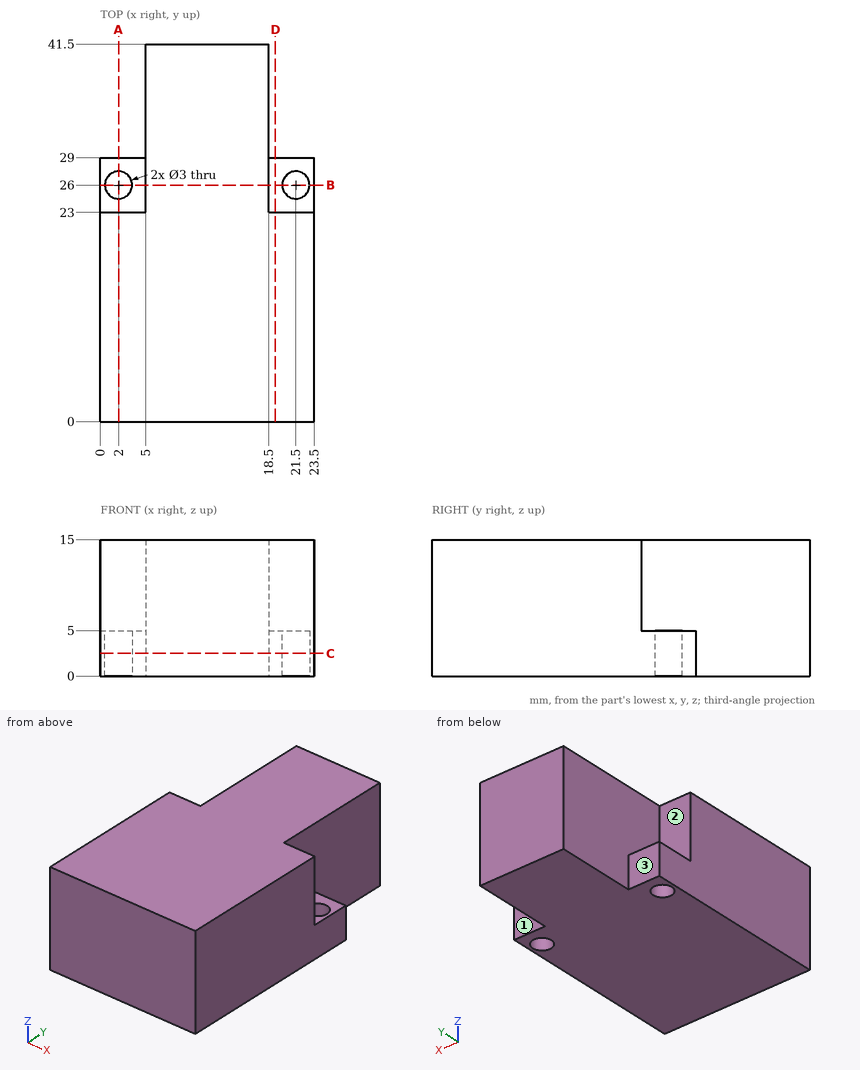
Print and shaded views of the part. All mm, measured from the part's lowest x, y and z. A direction names the side the tool comes from. Give positions to 0.01 mm unless a question says otherwise; leave off trailing zeros. Order: outer loops, then holes, each group sorted by start corner. A loop starts at its lowest first (then second) coordinate and runs counter-clockwise, first axis right, second up. Notation, with made-up numbers: (-39.75, 3.5) -> (5.25, 3.5) arc R20 cw to (5.25, 9.5) -> close; hole circle Ø7 at (40.25, 69.5). An arc over 180 degrees is marked (long way). Use CSV: the item, a comma, the result in double quotes.
1. Band-saw the part on B-B, the plane y = 26. Give the cut face in (x, z), then the cut area to 4 significant figures.
Outcome:
outline,"(0, 0) -> (0.5, 0) -> (0.5, 5) -> (0, 5) -> close; (3.5, 0) -> (20, 0) -> (20, 5) -> (18.5, 5) -> (18.5, 15) -> (5, 15) -> (5, 5) -> (3.5, 5) -> close; (23, 0) -> (23.5, 0) -> (23.5, 5) -> (23, 5) -> close"
area,"222.5 mm²"
2. Band-saw the part on A-A, the plane x = 2. Give the cut face in (y, z).
Outcome:
outline,"(0, 0) -> (24.5, 0) -> (24.5, 5) -> (23, 5) -> (23, 15) -> (0, 15) -> close; (27.5, 0) -> (29, 0) -> (29, 5) -> (27.5, 5) -> close"
3. Band-saw the part on C-C, the plane z = 2.5. Give the cut face in (x, y).
Outcome:
outline,"(0, 0) -> (23.5, 0) -> (23.5, 29) -> (18.5, 29) -> (18.5, 41.5) -> (5, 41.5) -> (5, 29) -> (0, 29) -> close; hole circle Ø3 at (2, 26); hole circle Ø3 at (21.5, 26)"
4. Band-saw the part on D-D, the plane x = 19.25. Give the cut face in (y, z).
Outcome:
outline,"(0, 0) -> (29, 0) -> (29, 5) -> (23, 5) -> (23, 15) -> (0, 15) -> close"
5. Drill centre lines: line 1 along Y through (x, z) = (21.5, 1.65); line 2 along X through (y, z) = (38, 13.5); line 3 along Y through (x, z) = (4.5, 14). Where is each one in solid material? Low to high. Write a range as from..to.
Outcome:
line 1,"0..24.5, 27.5..29"
line 2,"5..18.5"
line 3,"0..23"
6. Drop flat-ended pins along their axis: pin 1 (2.5 mm diameter, centred on x = 2.5, z = 10.5, fed in from +Y); pin 2 (1.5 mm diameter, centred on x = 20, y = 27.5, fed in from +Z); pin 3 (4 mm diameter, centred on x = 2.5, z = 1.5, fed in from +Y). Give the stop position or say it passes through.
Outcome:
pin 1,"y = 23"
pin 2,"z = 5"
pin 3,"y = 29"
7. 3-axis set-ups, long thin cutter, end or side, ignore diameter. For the marked faces 1, 2 and 3: which of +Z, -Z, +X, -X, +Y, -Y reach the whole face in a straight line?
Outcome:
face 1,"+Z, -Z, +X, +Y"
face 2,"+Z, -X, +Y"
face 3,"+Z, -Z, -X, +Y"
